```python
from build123d import *

# Parameters (mm, degrees)
DODANIE_WYCI_GNI_CIE1_DEPTH = 1


with BuildPart() as part:
    # Szkic1 → Dodanie-wyciągnięcie1 (new body)
    with BuildSketch(Plane.XY):
        with BuildLine():
            Line((0, 0), (0, 12))
            Line((0, 12), (58.245735195, 12))
            ThreePointArc((58.245735195, 12), (66.905989232, 17), (66.905989232, 27))
            Line((66.905989232, 27), (52.973720558, 51.131397208))
            Line((52.973720558, 51.131397208), (70.294228634, 61.131397208))
            Line((70.294228634, 61.131397208), (97.794228634, 13.5))
            ThreePointArc((97.794228634, 13.5), (97.794228634, 4.5), (90, 0))
            Line((90, 0), (0, 0))
        make_face()
    extrude(amount=DODANIE_WYCI_GNI_CIE1_DEPTH)


solid = part.part
```
For this review, take the finished solid that the model builds, in its own axes (mm). Give positions to 0.01 mm unless a question says otherwise; leave off trailing zeros. Write each loop counter-clockwise with the first axis right and the second up, starting at its lowest first coordinate (ties: lowest second). Pieces come first, ordered by that corner, then holes.
Item 1: Take a section at B-B (x = 35). Give the boundary of the cut face in (y, z).
Item 2: The part is to be moulded in two halves that separate along Y. For faces 1 (the face through (61, 11, 1)), 2 (the face through (60.037, 38.897, 0.493)), 3 (the face through (61.51, 56.06, 0.49)), say which applies: +Y half, -Y half, draft (parallel to the pull), parting line (faces both ways), or undercut.
Item 3: Wall thickness on probe 1 along Y at (x, z) = (24.5, 0.75); probe 2 along Y at (x, z) = (59, 0.35); probe 3 along X at (y, z) = (40, 0.1): over which ranges is each line inside the solid? List them lowest first.
Item 4: Take a section at A-A (z = 0.2). Give the boundary of the cut face in (x, y).
Item 5: Insertion check: P1, Ø0.5, axis at x = 15.5, z = 0.5, coming from the +Y side. The pin has a flat end and moves straight along its axis. Give the tip position at first contact, or say it passes through.
Item 6: Take a section at C-C (y = 33.5). Give the boundary of the cut face in (x, z), and give its area (3 significant figures).
Established:
1. outline: (0, 0) - (12, 0) - (12, 1) - (0, 1) - close
2. face 1: draft
2. face 2: undercut
2. face 3: +Y half
3. probe 1: y = 0 to 12
3. probe 2: y = 0 to 12.03, 40.69 to 54.61
3. probe 3: x = 59.4 to 82.49
4. outline: (0, 0) - (90, 0) arc R9 ccw to (97.79, 13.5) - (70.29, 61.13) - (52.97, 51.13) - (66.91, 27) arc R10 cw to (58.25, 12) - (0, 12) - close
5. P1: stops at y = 12
6. outline: (63.15, 0) - (86.25, 0) - (86.25, 1) - (63.15, 1) - close
6. area: 23.1 mm2
